Part model, mm, in its own coordinate system. A direction names the side the tool comes from. Coordinates: 2 decimals unless noted, no trailing zeros. Loops run counter-clockwise (first coordinate to the right, second up) from the corner with the lowest first, then second, coordinate; pieces in that order, holes last. Notation, with made-up numbers: (-33, 31) - (5, 31) arc R14 cw to (5, 36) - close; hole circle Ø3 at (-6.5, 38). An arc over 180 degrees is marked (long way). Use a Markdown table: item, result. Add a question column.
1. 3-axis set-ups, long thin cutter, end or side, ignore diameter. For faces 1 (the flat face through (-45, -16, -73)), 2 (the cylindrical face through (-10.955, -8.112, 83.434)): which of +Z, -Z, +X, -X, +Y, -Y reach the whole face in a straight line?
2. Drop flat-ended pins along their axis: pin 1 (4 mm diameter, centred on x = 77.5, y = 3.5, fed in from +Z); pin 2 (4 mm diameter, centred on y = 10.5, z = 56, fed in from -X); pin 3 (1.5 mm diameter, centred on y = 1.5, z = -76, fed in from +X). Give the stop position or say it passes through.
3. Band-saw the part on A-A, the plane z = 0. Give the cut face in (x, y), plus the area to 3 significant figures.
4. Band-saw the part on C-C, the plane y = 9. Give the cut face in (x, z), plus the area to 3 significant figures.
5. Band-saw the part on D-D, the plane x = 80. Give the cut face in (y, z), plus the area to 3 significant figures.
6. Wall check: probe 1 along Z at (x, y) = (0, -12.5); probe 2 along Z at (x, y) = (0, 11.5); probe 3 along Y at (x, z) = (63, 49). Give the ranges that are in metal, low to high. Write a range as [from, to].
7. Band-saw the part on B-B, the plane x = 0. Give the cut face in (y, z).
8. Pull direction Z, two halves, no side cores. Call faces 3 (the cylindrical face through (73.145, 21.199, 23.035)), 4 (the cylindrical face through (-18.142, 28.297, -81.696)), 5 (the flat face through (-67, 14, -51)): pulls with the +Z half, pulls with the -Z half, needs draft (parallel to the pull), parting line crosses it, or undercut.
from build123d import *

# Parameters (mm, degrees)
F0_R     = 98.686434
F0_R_2   = 83.686432
F1_DEPTH = 16
F0_R_3   = 76.686434
F2_DEPTH = 14
F3_DEPTH = 43
F4_R     = 84.150337
F4_R_2   = 83.686432
F5_DEPTH = 16
F6_R     = 99.162904
F6_R_2   = 98.686434
F7_DEPTH = 30


with BuildPart() as f1:
    # F0 (on Front) → F1 (new body)
    with BuildSketch(Plane.XZ):
        Circle(F0_R)
        Circle(F0_R_2, mode=Mode.SUBTRACT)
    extrude(amount=F1_DEPTH)

    # F0 (on Front) → F2 (join)
    with BuildSketch(Plane.XZ):
        Circle(F0_R_2)
        Circle(F0_R_3, mode=Mode.SUBTRACT)
        Circle(F0_R)
        Circle(F0_R_2, mode=Mode.SUBTRACT)
    extrude(amount=-F2_DEPTH)

    # F0 (on Front) → F3 (join)
    with BuildSketch(Plane.XZ):
        Circle(F0_R_2)
        Circle(F0_R_3, mode=Mode.SUBTRACT)
    extrude(amount=-F3_DEPTH)

    # F4 (on face) → F5 (cut)
    with BuildSketch(Plane.XZ.offset(16)):
        Circle(F4_R)
        Circle(F4_R_2, mode=Mode.SUBTRACT)
    extrude(amount=-F5_DEPTH, mode=Mode.SUBTRACT)

    # F6 (on face) → F7 (join)
    with BuildSketch(Plane.XZ.offset(16)):
        Circle(F6_R)
        Circle(F6_R_2, mode=Mode.SUBTRACT)
    extrude(amount=-F7_DEPTH)


solid = f1.part
Geometry check:
| question | item | result |
|---|---|---|
| 1 | face 1 | +Z, -Z, +X, -X, -Y |
| 1 | face 2 | -Y |
| 2 | pin 1 | stops at z = 64.29 |
| 2 | pin 2 | stops at x = -83.17 |
| 2 | pin 3 | stops at x = 64.58 |
| 3 | outline | (-99.16, -16) - (-84.15, -16) - (-84.15, 0) - (-76.69, 0) - (-76.69, 43) - (-83.69, 43) - (-83.69, 14) - (-99.16, 14) - close; (76.69, 0) - (84.15, 0) - (84.15, -16) - (99.16, -16) - (99.16, 14) - (83.69, 14) - (83.69, 43) - (76.69, 43) - close |
| 3 | area | 1,520 mm^2 |
| 4 | outline | circle Ø198.33 at (0, 0); hole circle Ø153.37 at (0, 0) |
| 4 | area | 12,400 mm^2 |
| 5 | outline | (-16, -58.59) - (14, -58.59) - (14, -24.56) - (43, -24.56) - (43, 24.56) - (14, 24.56) - (14, 58.59) - (-16, 58.59) - (-16, 26.1) - (0, 26.1) - (0, -26.1) - (-16, -26.1) - close |
| 5 | area | 4,110 mm^2 |
| 6 | probe 1 | z = [-99.16, -84.15], [84.15, 99.16] |
| 6 | probe 2 | z = [-99.16, -76.69], [76.69, 99.16] |
| 6 | probe 3 | y = [0, 43] |
| 7 | outline | (-16, -99.16) - (14, -99.16) - (14, -83.69) - (43, -83.69) - (43, -76.69) - (0, -76.69) - (0, -84.15) - (-16, -84.15) - close; (-16, 84.15) - (0, 84.15) - (0, 76.69) - (43, 76.69) - (43, 83.69) - (14, 83.69) - (14, 99.16) - (-16, 99.16) - close |
| 8 | face 3 | undercut |
| 8 | face 4 | parting line crosses it |
| 8 | face 5 | needs draft |
